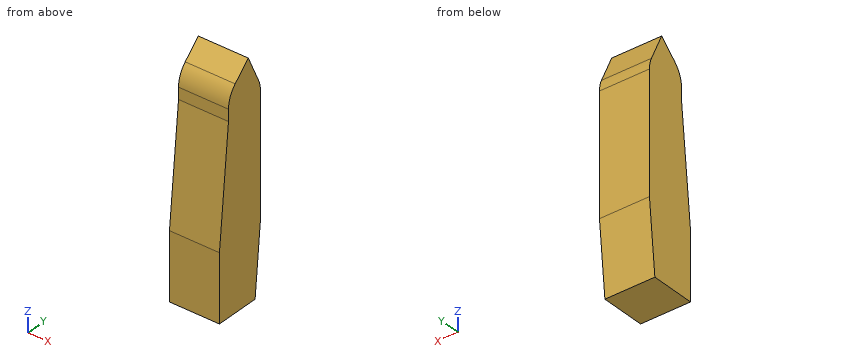
from build123d import *

# Parameters (mm, degrees)
F0_W     = 9.3000009656
F0_H     = 9.5999985933
F1_DEPTH = 43
F3_DEPTH = 9.3010009656
F4_R     = 5


with BuildPart() as f1:
    # F0 (on Top) → F1 (new body)
    with BuildSketch(Plane.XY):
        with Locations((-54.4500015676, 53.8500025868)):
            Rectangle(F0_W, F0_H)
    extrude(amount=F1_DEPTH)

    # F2 (on face) → F3 (cut, through all)
    with BuildSketch(Plane(origin=(-59.1000020504, 0, 0), x_dir=(0, -1, 0), z_dir=(-1, 0, 0))):
        Polygon((-49.0500032902, 43), (-55.7899177074, 43), (-51.1679239571, 38.6058986187), (-51.1679239571, 34.302663058), (-49.0500032902, 12.4677242711), align=None)
        Polygon((-58.6500018835, 36.8527285755), (-55.7899177074, 43), (-58.6500018835, 43), align=None)
        Polygon((-57.3837086558, 0), (-58.6500018835, 13.4239988402), (-58.6500018835, 0), align=None)
    extrude(amount=-F3_DEPTH, mode=Mode.SUBTRACT)

    # F4
    f4_edges = [f1.edges().sort_by_distance(p)[0] for p in [
        (-54.450002, 51.167924, 38.605899),
        (-54.450002, 58.650002, 36.852729),
    ]]
    fillet(f4_edges, radius=F4_R)


solid = f1.part
Work out the finished part from the listing and answer in its coordinate system (mm). Give positions to 0.01 mm unless a question says otherwise; leave off trailing zeros. Write each loop counter-clockwise with the first axis right and the second up, starting at its lowest first coordinate (ties: lowest second). Pieces come first, ordered by that corner, then holes. Notation, with made-up numbers: M -30.5,84 L -16.5,84 A13 ccw -16.5,91 Z; hole C 69.25,-4.5 d11. An arc over 180 degrees is marked long. Answer as CSV lines item,"result".
Q1. A cutting plane is placed at B-B on z = 5.5. Write down the section's boundary in (x, y).
A:
outline,"M -59.1,49.05 L -49.8,49.05 L -49.8,57.9 L -59.1,57.9 Z"
Q2. A cutting plane is placed at C-C on y = 53.5. Write down the section's boundary in (x, z), plus the area to 3 significant figures.
A:
outline,"M -59.1,0 L -49.8,0 L -49.8,40.82 L -59.1,40.82 Z"
area,"380 mm²"
Q3. Find the intervals of material crossed by probe 1 along Y at (x, z) = (-54.5, 35.5); probe 2 along Y at (x, z) = (-51.5, 8); probe 3 along Z at (x, y) = (-51, 52.25), in increasing order. Write a range as [from, to].
A:
probe 1,"y = [51.17, 58.65]"
probe 2,"y = [49.05, 58.14]"
probe 3,"z = [0, 39.57]"
Q4. A cutting plane is placed at A-A on x = -54.25. Write down the section's boundary in (y, z), plus the area to 3 significant figures.
A:
outline,"M 49.05,0 L 57.38,0 L 58.65,13.42 L 58.65,35.75 A5 ccw 58.18,37.86 L 55.79,43 L 52.72,40.08 A5 ccw 51.17,36.46 L 51.17,34.3 L 49.05,12.47 Z"
area,"343 mm²"
Q5. Given P1, Ø1.1, axis at x = -53.5, z = 35.5, coming from the -Y side, flat-ended and moving along its own axis, determine where the tip first touches the part or whether it passes through.
A:
P1,"stops at y = 51.17"
